Source: three-view drawing plus pictorial views. Frame: mm from the lowest corner of the part. Give positions to 0.01 mm unless a question says otherwise; leave off trailing zeros. Order: outer loops, then holes, each group sorted by start corner. A loop starts at its lowest first (then second) coordinate and runs counter-clockwise, first axis right, second up. Notation, with made-up numbers: (56, 65) - (95, 65) arc R13 cw to (95, 83) - close; hole circle Ø2 at (87.5, 11). An arc over 180 degrees is marked (long way). Use CSV: the item, a comma, the result in double quotes.
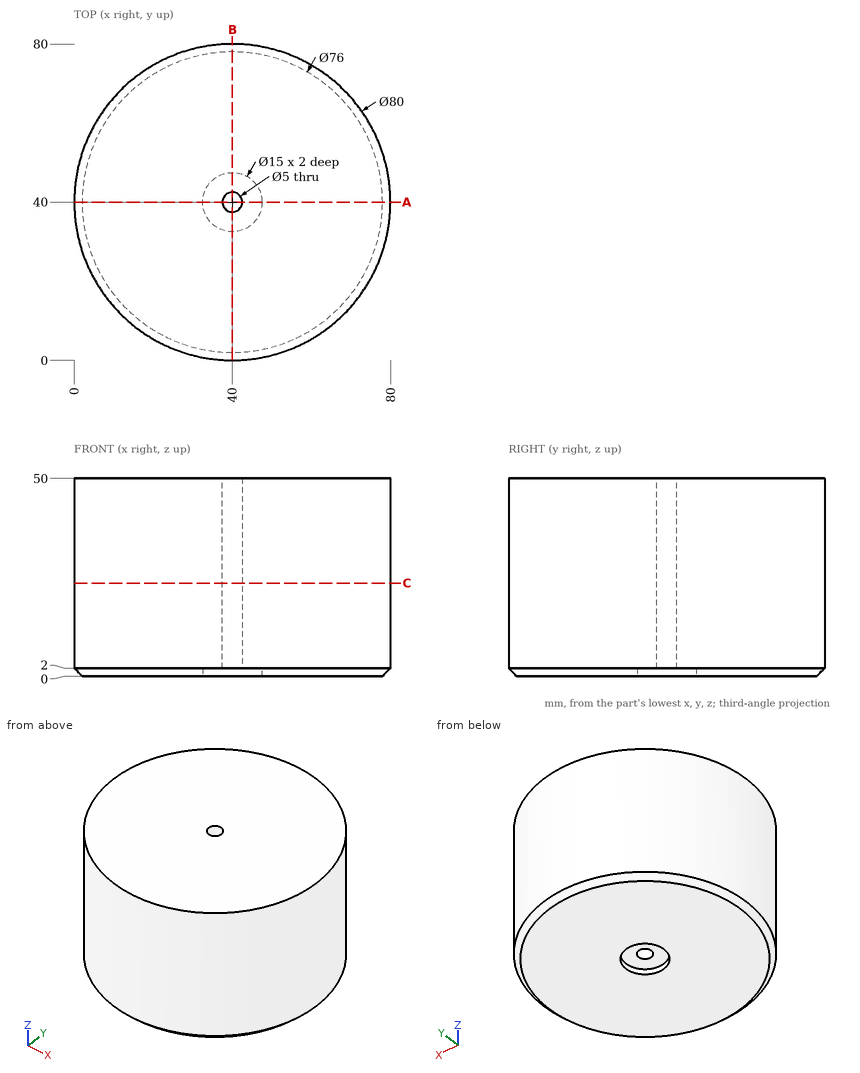
Item 1: Section C-C on z = 23.5. Return the cut outline in (x, y).
Filled in:
outline,"circle Ø80 at (40, 40); hole circle Ø5 at (40, 40)"
Item 2: Material intervals for line 1 (Y direction, x = 40, z = 37.5); line 2 (Y direction, x = 41, z = 9.5), sorted ascending. Write a range as from..to.
Filled in:
line 1,"y = 0..37.5, 42.5..80"
line 2,"y = 0.01..37.71, 42.29..79.99"
Item 3: First-contact query: pin 1 (12 mm diameter, centred on x = 29.5, z = 22, fed in from -Y); pin 2 (5 mm diameter, centred on x = 39, z = 39.5, fed in from +Y); pin 3 (3 mm diameter, centred on x = 52, z = 41, fed in from +Y); pin 4 (2 mm diameter, centred on x = 37.5, y = 9, fed in from -Z). Flat tips, straight axial feed; report the tip coordinate or a pass-through.
Filled in:
pin 1,"stops at y = 0.25"
pin 2,"stops at y = 80"
pin 3,"stops at y = 78.6"
pin 4,"stops at z = 0"
Item 4: Section A-A on y = 40. Return the cut outline in (x, z), then the cut area to 3 significant figures.
Filled in:
outline,"(0, 2) - (2, 0) - (32.5, 0) - (32.5, 2) - (37.5, 2) - (37.5, 50) - (0, 50) - close; (42.5, 2) - (47.5, 2) - (47.5, 0) - (78, 0) - (80, 2) - (80, 50) - (42.5, 50) - close"
area,"3,730 mm2"
